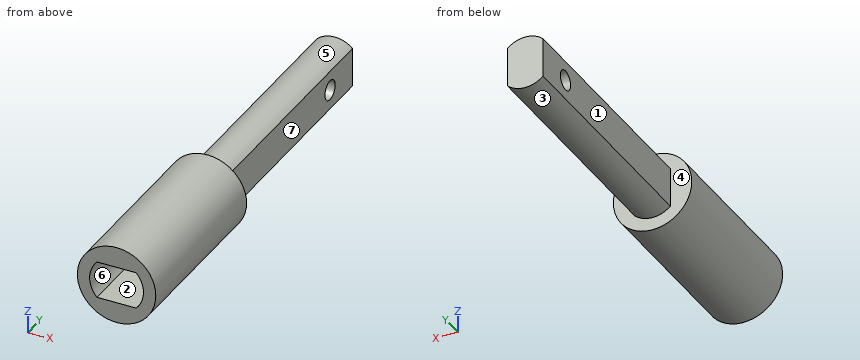
```python
from build123d import *

# Parameters (mm, degrees)
SKETCH1_R           = 4
BOSS_EXTRUDE1_DEPTH = 9
SKETCH2_R           = 4
BOSS_EXTRUDE2_DEPTH = 8.83
BOSS_EXTRUDE3_DEPTH = 25
SKETCH4_R           = 1
CUT_EXTRUDE1_DEPTH  = 25


with BuildPart() as part:
    # Sketch1 → Boss-Extrude1 (new body)
    with BuildSketch(Plane(origin=(0, 0, 0), x_dir=(1, 0, 0), z_dir=(0, 1, 0))):
        Circle(SKETCH1_R)
        with BuildLine():
            Line((-2, 1.887458609), (2, 1.887458609))
            ThreePointArc((2, 1.887458609), (2.75, 0), (2, -1.887458609))
            Line((2, -1.887458609), (-2, -1.887458609))
            ThreePointArc((-2, -1.887458609), (-2.75, 0), (-2, 1.887458609))
        make_face(mode=Mode.SUBTRACT)
    extrude(amount=BOSS_EXTRUDE1_DEPTH)

    # Sketch2 → Boss-Extrude2 (add)
    with BuildSketch(Plane(origin=(0, 9, 0), x_dir=(1, 0, 0), z_dir=(0, 1, 0))):
        Circle(SKETCH2_R)
    extrude(amount=BOSS_EXTRUDE2_DEPTH)

    # Sketch3 → Boss-Extrude3 (add)
    with BuildSketch(Plane(origin=(0, 17.83, 0), x_dir=(1, 0, 0), z_dir=(0, 1, 0))):
        with BuildLine():
            Line((1.813835715, 2), (1.813835715, -2))
            ThreePointArc((1.813835715, -2), (0, -2.7), (-1.813835715, -2))
            Line((-1.813835715, -2), (-1.813835715, 2))
            ThreePointArc((-1.813835715, 2), (0, 2.7), (1.813835715, 2))
        make_face()
    extrude(amount=BOSS_EXTRUDE3_DEPTH)

    # Sketch4 → Cut-Extrude1 (cut)
    with BuildSketch(Plane(origin=(1.813835715, 0, 0), x_dir=(0, 0, -1), z_dir=(1, 0, 0))):
        with Locations((0, 38.421822436)):
            Circle(SKETCH4_R)
    extrude(amount=-CUT_EXTRUDE1_DEPTH, mode=Mode.SUBTRACT)


solid = part.part
```
For this review, take the finished solid that the model builds, in its own axes (mm). Face numbers are marked on the shaded views. A direction names the side the tool comes from. Coordinates: 2 decimals unless noted, no trailing zeros. Write each loop counter-clockwise with the first axis right and the second up, starting at its lowest first coordinate (ties: lowest second). Pieces come first, ordered by that corner, then holes. Notation, with made-up numbers: (-33.5, 8.25) - (9.5, 8.25) arc R20 ccw to (9.5, 33.25) - close; hole circle Ø9 at (-4.75, -14.75). An arc over 180 degrees is marked (long way). Put each result on its own line as item: value.
1. Add section D-D, the plane x = -3.5. Give the boundary of the cut face in (y, z), then the cut area to 3 significant figures.
Values found:
outline: (0, -1.94) - (17.83, -1.94) - (17.83, 1.94) - (0, 1.94) - close
area: 69.1 mm²
2. Add section A-A, the plane z = 0. Give the boundary of the cut face in (x, y), then the cut area to 3 significant figures.
Values found:
outline: (-4, 0) - (-2.75, 0) - (-2.75, 9) - (2.75, 9) - (2.75, 0) - (4, 0) - (4, 17.83) - (1.81, 17.83) - (1.81, 37.42) - (-1.81, 37.42) - (-1.81, 17.83) - (-4, 17.83) - close; (-1.81, 39.42) - (1.81, 39.42) - (1.81, 42.83) - (-1.81, 42.83) - close
area: 177 mm²
3. Add section C-C, the plane y = 12. Give the boundary of the cut face in (x, z), then the cut area to 3 significant figures.
Values found:
outline: circle Ø8 at (0, 0)
area: 50.3 mm²
4. Wall thickness on probe 1 along Y at (x, z) = (0.8, 0); probe 2 along Y at (x, z) = (3, 1.5); probe 3 along Y at (x, z) = (-1.5, -0.5): over which ranges is each line inside the solid? List them lowest first.
Values found:
probe 1: 9 to 37.42, 39.42 to 42.83
probe 2: 0 to 17.83
probe 3: 9 to 37.56, 39.29 to 42.83
5. Mouldability with a two-part tool opening along Z and no side actions: class the marked faces 5, 6 and 7 as released by +Z, released by -Z, zero draft, split by the parting line, or undercut.
Values found:
face 5: released by +Z
face 6: undercut
face 7: zero draft
6. Machinability: for the marked faces 1, 2, 3 and 4, which of the approach directions +Z, -Z, +X, -X, +Y, -Y give a long, thin tool a straight path to every point of the face, cutting with its end or side? Answer none if there is none.
Values found:
face 1: +Z, -Z, -X, +Y
face 2: -Y
face 3: -Z, +Y
face 4: +Y
7. Add section B-B, the plane x = 0. Give the boundary of the cut face in (y, z), then the cut area to 3 significant figures.
Values found:
outline: (0, -4) - (17.83, -4) - (17.83, -2.7) - (42.83, -2.7) - (42.83, 2.7) - (17.83, 2.7) - (17.83, 4) - (0, 4) - (0, 1.89) - (9, 1.89) - (9, -1.89) - (0, -1.89) - close; hole circle Ø2 at (38.42, 0)
area: 241 mm²
8. For pin 1 (1.9 mm diameter, centred on x = 0, z = -0.5, fed in from -Y); pin 2 (1 mm diameter, centred on x = -0.5, z = 2, fed in from -Y); pin 3 (3 mm diameter, centred on y = 38.42, z = 0, fed in from +X); pin 4 (4.5 mm diameter, centred on y = 31, z = 1, fed in from -X), all flat-tipped, find the tip position at first contact; note any pin that passes through.
Values found:
pin 1: y = 9
pin 2: y = 0
pin 3: x = 1.81
pin 4: x = -1.81
